Source: CAD feature listing. Evaluate the final solid. Frame: model axes, mm. Give positions to 0.01 mm unless a question says otherwise; leave off trailing zeros. Write each loop counter-clockwise with the first axis right and the second up, starting at its lowest first coordinate (ties: lowest second). Pieces come first, ordered by that corner, then holes. Notation, with made-up numbers: M -28,11 L 28,11 A20 ccw 28,38 Z; hole C 77.25,-12.75 d5. An arc over 180 degrees is marked long. Return JSON: item names as keys, results as strings.
```python
from build123d import *

# Parameters (mm, degrees)
SKETCH1_W                        = 30
SKETCH1_H                        = 54
PLATE_54X30_DEPTH                = 2
OPTICAL_WINDOW_10X10_START       = -0.1
SKETCH2_W                        = 10
SKETCH2_H                        = 10
OPTICAL_WINDOW_10X10_DEPTH       = 2.2
VERTICAL_M3_ADJUSTMENT_1_START   = -0.1
SKETCH3_W                        = 10
SKETCH3_H                        = 3.4
VERTICAL_M3_ADJUSTMENT_1_DEPTH   = 2.2
SKETCH4_W                        = 10
SKETCH4_H                        = 3.4
VERTICAL_M3_ADJUSTMENT_1_2_DEPTH = 2.2


with BuildPart() as part:
    # Sketch1 → Plate_54x30 (new body)
    with BuildSketch(Plane.XY):
        Rectangle(SKETCH1_W, SKETCH1_H)
    extrude(amount=PLATE_54X30_DEPTH)

    # Sketch2 → Optical_Window_10x10 (cut)
    with BuildSketch(Plane.XY.offset(OPTICAL_WINDOW_10X10_START)):
        Rectangle(SKETCH2_W, SKETCH2_H)
    extrude(amount=OPTICAL_WINDOW_10X10_DEPTH, mode=Mode.SUBTRACT)

    # Sketch3 → Vertical_M3_Adjustment_-1 (cut)
    with BuildSketch(Plane.XY.offset(VERTICAL_M3_ADJUSTMENT_1_START)):
        with Locations((0, -22)):
            Rectangle(SKETCH3_W, SKETCH3_H)
    extrude(amount=VERTICAL_M3_ADJUSTMENT_1_DEPTH, mode=Mode.SUBTRACT)

    # Sketch4 → Vertical_M3_Adjustment_1 2 (cut)
    with BuildSketch(Plane.XY.offset(VERTICAL_M3_ADJUSTMENT_1_START)):
        with Locations((0, 22)):
            Rectangle(SKETCH4_W, SKETCH4_H)
    extrude(amount=VERTICAL_M3_ADJUSTMENT_1_2_DEPTH, mode=Mode.SUBTRACT)


solid = part.part
```
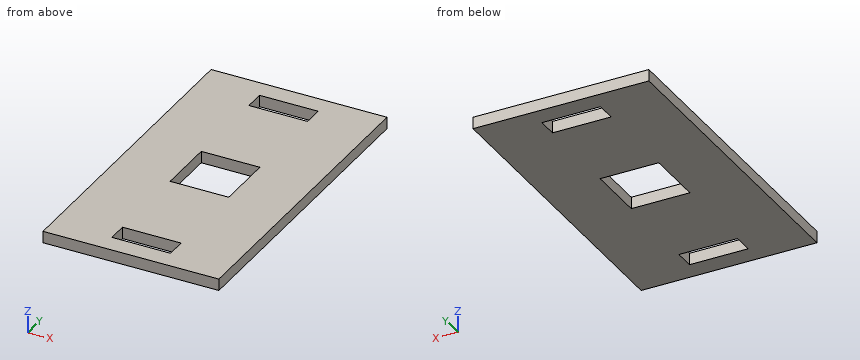
1) Line query: line 1 (Y direction, x = -4.75, z = 1.8); line 2 (X direction, y = 22, z = 1.55). Output: solid intervals per line, ascending. Write a range as [from, to].
Numbers:
{"line 1": "y = [-27, -23.7], [-20.3, -5], [5, 20.3], [23.7, 27]", "line 2": "x = [-15, -5], [5, 15]"}
2) Cut plane C-C, the plane y = 21. Return the cut outline in (x, z).
Numbers:
{"outline": "M -15,0 L -5,0 L -5,2 L -15,2 Z; M 5,0 L 15,0 L 15,2 L 5,2 Z"}
3) Cut plane B-B, the plane z = 0.85. Return the cut outline in (x, y), then the cut area to 3 significant figures.
Numbers:
{"outline": "M -15,-27 L 15,-27 L 15,27 L -15,27 Z; hole M -5,-23.7 L 5,-23.7 L 5,-20.3 L -5,-20.3 Z; hole M -5,-5 L 5,-5 L 5,5 L -5,5 Z; hole M -5,20.3 L 5,20.3 L 5,23.7 L -5,23.7 Z", "area": "1,450 mm²"}
4) Cut plane A-A, the plane x = 3. Return the cut outline in (y, z), then the cut area to 3 significant figures.
Numbers:
{"outline": "M -27,0 L -23.7,0 L -23.7,2 L -27,2 Z; M -20.3,0 L -5,0 L -5,2 L -20.3,2 Z; M 5,0 L 20.3,0 L 20.3,2 L 5,2 Z; M 23.7,0 L 27,0 L 27,2 L 23.7,2 Z", "area": "74.4 mm²"}
